```python
from build123d import *

# Parameters (mm, degrees)
SKETCH1_R            = 33
SKETCH1_R_2          = 15.25
BOSS_EXTRUDE1_DEPTH  = 4
SKETCH2_R            = 18.25
SKETCH2_R_2          = 15.25
BOSS_EXTRUDE2_DEPTH  = 13.5
SKETCH3_R            = 18.25
SKETCH3_R_2          = 8.25
BOSS_EXTRUDE3_DEPTH  = 3
M3_CLEARANCE_HOLE2_D = 3.2
CUT_EXTRUDE2_DEPTH   = 7
SKETCH10_R           = 35
CUT_EXTRUDE3_DEPTH   = 1
M4_CLEARANCE_HOLE1_D = 4.3
FILLET1_R            = 0.5
FILLET2_R            = 0.5
SKETCH13_R           = 30
CUT_EXTRUDE4_DEPTH   = 1
FILLET3_R            = 0.5


with BuildPart() as part:
    # Sketch1 → Boss-Extrude1 (new body)
    with BuildSketch(Plane.XY):
        Circle(SKETCH1_R)
        Circle(SKETCH1_R_2, mode=Mode.SUBTRACT)
    extrude(amount=BOSS_EXTRUDE1_DEPTH)

    # Sketch2 → Boss-Extrude2 (add)
    with BuildSketch(Plane.XY.offset(4)):
        Circle(SKETCH2_R)
        Circle(SKETCH2_R_2, mode=Mode.SUBTRACT)
    extrude(amount=BOSS_EXTRUDE2_DEPTH)

    # Sketch3 → Boss-Extrude3 (add)
    with BuildSketch(Plane.XY.offset(17.5)):
        Circle(SKETCH3_R)
        Circle(SKETCH3_R_2, mode=Mode.SUBTRACT)
    extrude(amount=-BOSS_EXTRUDE3_DEPTH)

    # M3 Clearance Hole2 (through all)
    with Locations(Plane.XY.offset(17.5)):
        with Locations((0, 11), (9.526279442, 5.5), (9.526279442, -5.5), (0, -11), (-9.526279442, -5.5), (-9.526279442, 5.5), (0, 0)):
            Hole(M3_CLEARANCE_HOLE2_D / 2)

    # Sketch9 → Cut-Extrude2 (cut)
    with BuildSketch(Plane.XY.offset(14.5)):
        with BuildLine():
            ThreePointArc((-12.688309019, 5.916655664), (-9.899494937, 9.899494937), (-5.916655664, 12.688309019))
            Line((-5.916655664, 12.688309019), (-7.712783277, 16.540117113))
            ThreePointArc((-7.712783277, 16.540117113), (-12.904698757, 12.904698757), (-16.540117113, 7.712783277))
            Line((-16.540117113, 7.712783277), (-12.688309019, 5.916655664))
        make_face()
        with BuildLine():
            Line((-7.712783277, -16.540117113), (-5.916655664, -12.688309019))
            ThreePointArc((-5.916655664, -12.688309019), (-9.899494937, -9.899494937), (-12.688309019, -5.916655664))
            Line((-12.688309019, -5.916655664), (-16.540117113, -7.712783277))
            ThreePointArc((-16.540117113, -7.712783277), (-12.904698757, -12.904698757), (-7.712783277, -16.540117113))
        make_face()
    extrude(amount=-CUT_EXTRUDE2_DEPTH, mode=Mode.SUBTRACT)

    # Sketch10 → Cut-Extrude3 (cut)
    with BuildSketch(Plane(origin=(0, 0, 0), x_dir=(-1, 0, 0), z_dir=(0, 0, -1))):
        Circle(SKETCH10_R)
    extrude(amount=-CUT_EXTRUDE3_DEPTH, mode=Mode.SUBTRACT)

    # M4 Clearance Hole1 (through all)
    with Locations(Plane.XY.offset(4)):
        with Locations((0, 25), (25, 0), (0, -25), (-25, 0), (0, 0)):
            Hole(M4_CLEARANCE_HOLE1_D / 2)

    # Fillet1
    fillet1_edges = [part.edges().sort_by_distance(p)[0] for p in [
        (-18.25, 0, 4),
        (-15.25, 0, 14.5),
    ]]
    fillet(fillet1_edges, radius=FILLET1_R)

    # Fillet2
    fillet2_edges = [part.edges().sort_by_distance(p)[0] for p in [
        (-15.25, 0, 1),
    ]]
    fillet(fillet2_edges, radius=FILLET2_R)

    # Sketch13 → Cut-Extrude4 (cut)
    with BuildSketch(Plane(origin=(0, 0, 1), x_dir=(-1, 0, 0), z_dir=(0, 0, -1))):
        Circle(SKETCH13_R)
    extrude(amount=-CUT_EXTRUDE4_DEPTH, mode=Mode.SUBTRACT)

    # Fillet3
    fillet3_edges = [part.edges().sort_by_distance(p)[0] for p in [
        (30, 0, 2),
    ]]
    fillet(fillet3_edges, radius=FILLET3_R)


solid = part.part
```
Design review of the part built by this model. Coordinates are the model's own, in mm. A direction names the side the tool comes from. Coordinates: 2 decimals unless noted, no trailing zeros. Loops run counter-clockwise (first coordinate to the right, second up) from the corner with the lowest first, then second, coordinate; pieces in that order, holes last.
Q1. For pin 1 (5 mm diameter, centred on x = 17.5, z = 15, fed in from +Y); pin 2 (5 mm diameter, centred on y = 4.5, z = 4.5, fed in from +X); pin 3 (2.5 mm diameter, centred on x = -9.53, y = 5.5, fed in from -Z); pin 4 (5.5 mm diameter, centred on x = 0, y = 25, fed in from +Z), all flat-tipped, find the tip position at first contact; note any pin that passes through.
Reported:
pin 1: stops at y = 10.4
pin 2: stops at x = 32.94
pin 3: passes through
pin 4: stops at z = 4
Q2. We need section B-B on x = 0. State how many separate pieces and enclosed holes the cut face has, and give its area (3 significant figures).
Reported:
separate pieces: 6
enclosed holes: 0
area: 164 mm2
Q3. Tool access review of faces 1 (the face through (-7.07, 15.16, 11.05)), 2 (the face through (-13, -13, 2)), 3 (the face through (-8, -3, 14.5)), 4 (the face through (-14.976, 6.984, 11.049)): name each direction out of +Z, -Z, +X, -X, +Y, -Y from which nothing blocks a thin tool from reaching the whole face with its end or side.
Reported:
face 1: -X
face 2: -Z
face 3: none
face 4: +Y
Q4. The part is to be moulded in two halves that separate along X. For faces 5 (the face through (17.4, 5.5, 10.9)), 6 (the face through (22.95, 0.65, 2.99)), 7 (the face through (14, -14, 4)), say which applies: +X half, -X half, draft (parallel to the pull), parting line (faces both ways), or undercut.
Reported:
face 5: parting line
face 6: undercut
face 7: draft
Q5. To check wall thickness, follow line 1 (Y direction, x = 0, z = 2.75); line 2 (Y direction, x = 0, z = 1.3); line 3 (Z direction, x = -12.5, y = -11.5). State the ranges of each line that lie inside material, in increasing order.
Reported:
line 1: y = -33 to -27.15, -22.85 to -15.25, 15.25 to 22.85, 27.15 to 33
line 2: y = -33 to -30, 30 to 33
line 3: z = 2 to 7.5, 14.5 to 17.5
Q6. We need section A-A on z = 12.25. State the section outline as (x, y) points, and give its area (3 significant figures).
Reported:
outline: (-16.54, -7.71) - (-13.82, -6.44) arc R15.25 cw to (-13.82, 6.44) - (-16.54, 7.71) arc R18.25 ccw to start; (-7.71, -16.54) arc R18.25 ccw (long way) to (-7.71, 16.54) - (-6.44, 13.82) arc R15.25 cw (long way) to (-6.44, -13.82) - close
area: 246 mm2
